from build123d import *

# Parameters (mm, degrees)
EXTRUDE_1_DEPTH     = 2
SKETCH_2_W          = 75
SKETCH_2_H          = 14
SKETCH_2_R          = 2.5
EXTRUDE_2_DEPTH     = 2
CUT_EXTRUDE_2_DEPTH = 39.20013089
FILLET_1_R          = 7


with BuildPart() as part:
    # 草图1 → 凸台-拉伸1 (new body)
    with BuildSketch(Plane.XY):
        with BuildLine():
            Line((-2.645751311, 3), (2.645751311, 3))
            ThreePointArc((2.645751311, 3), (4, 0), (2.645751311, -3))
            Line((2.645751311, -3), (-2.645751311, -3))
            ThreePointArc((-2.645751311, -3), (-4, 0), (-2.645751311, 3))
        make_face()
    extrude(amount=EXTRUDE_1_DEPTH)

    # 草图2 → 凸台-拉伸2 (add)
    with BuildSketch(Plane.XY.offset(2)):
        Rectangle(SKETCH_2_W, SKETCH_2_H)
        with Locations((-30, 0)):
            Circle(SKETCH_2_R, mode=Mode.SUBTRACT)
        with Locations((30, 0)):
            Circle(SKETCH_2_R, mode=Mode.SUBTRACT)
    extrude(amount=-EXTRUDE_2_DEPTH)

    # 草图3 → 切除-拉伸2 (cut, through all)
    with BuildSketch(Plane.XY):
        with BuildLine():
            Line((-2.645751311, 3), (2.645751311, 3))
            ThreePointArc((2.645751311, 3), (4, 0), (2.645751311, -3))
            Line((2.645751311, -3), (-2.645751311, -3))
            ThreePointArc((-2.645751311, -3), (-4, 0), (-2.645751311, 3))
        make_face()
    extrude(amount=CUT_EXTRUDE_2_DEPTH, mode=Mode.SUBTRACT)

    # 圆角1
    fillet_1_edges = [part.edges().sort_by_distance(p)[0] for p in [
        (37.5, -7, 1),
        (37.5, 7, 1),
        (-37.5, -7, 1),
        (-37.5, 7, 1),
    ]]
    fillet(fillet_1_edges, radius=FILLET_1_R - 0.0001)  # a hair under: the kernel refuses the full size


solid = part.part
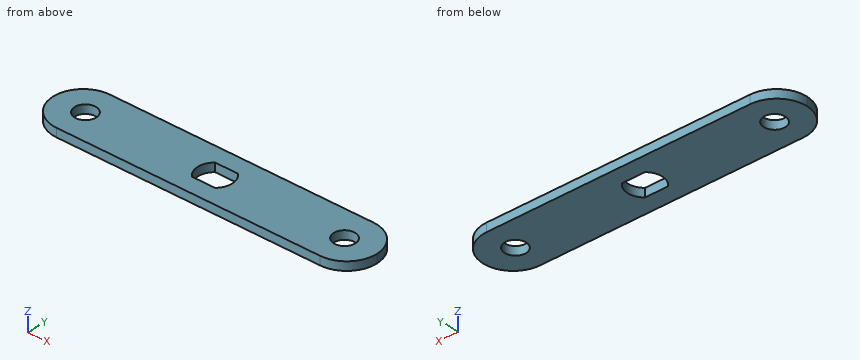
For this review, take the finished solid that the model builds, in its own axes (mm). Give positions to 0.01 mm unless a question says otherwise; leave off trailing zeros. Order: outer loops, then holes, each group sorted by start corner. A loop starts at its lowest first (then second) coordinate and runs counter-clockwise, first axis right, second up. Notation, with made-up numbers: (25, -15.75) - (54, -15.75) arc R16 cw to (54, 5.25) - close; hole circle Ø7 at (-38, 86.25). An arc over 180 degrees is marked (long way). Answer as a JSON object with one key per item and string values. Group by question number.
Item 1: Take a section at D-D on y = 5.5. Give the boundary of the cut face in (x, z), and give its area (3 significant figures).
Item 2: Take a section at C-C on x = -29. Give the boundary of the cut face in (y, z).
Item 3: Take a section at B-B on z = 1.45. Give the number of separate pieces and of enclosed holes in the cut face, and give its area (3 significant figures).
Item 4: Take a section at A-A on y = -0.75. Give the boundary of the cut face in (x, z), and give its area (3 significant figures).
Item 5: Wall thickness on line 1 along Y through (x, z) = (-30, 1.55); line 2 along X through (y, z) = (-1, 0.55); line 3 along X through (y, z) = (2, 0.1): over which ranges is each line inside the solid? List them lowest first.
Reported:
{
 "1": {"outline": "(-34.83, 0) - (34.83, 0) - (34.83, 2) - (-34.83, 2) - close", "area": "139 mm^2"},
 "2": {"outline": "(-7, 0) - (-2.29, 0) - (-2.29, 2) - (-7, 2) - close; (2.29, 0) - (7, 0) - (7, 2) - (2.29, 2) - close"},
 "3": {"separate pieces": "1", "enclosed holes": "3", "area": "926 mm^2"},
 "4": {"outline": "(-37.46, 0) - (-32.38, 0) - (-32.38, 2) - (-37.46, 2) - close; (-27.62, 0) - (-3.93, 0) - (-3.93, 2) - (-27.62, 2) - close; (3.93, 0) - (27.62, 0) - (27.62, 2) - (3.93, 2) - close; (32.38, 0) - (37.46, 0) - (37.46, 2) - (32.38, 2) - close", "area": "115 mm^2"},
 "5": {"line 1": "-7 to -2.5, 2.5 to 7", "line 2": "-37.43 to -32.29, -27.71 to -3.87, 3.87 to 27.71, 32.29 to 37.43", "line 3": "-37.21 to -31.5, -28.5 to -3.46, 3.46 to 28.5, 31.5 to 37.21"}
}
